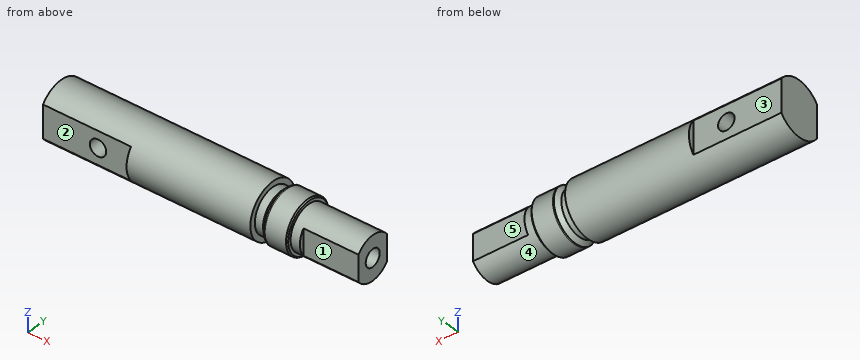
```python
from build123d import *

# Parameters (mm, degrees)
CUT_EXTRUDE1_START               = -16
CUT_EXTRUDE1_DEPTH               = 16
F_3_0MM_DOWEL_HOLE1_D            = 3
CUT_EXTRUDE3_START               = -20
SKETCH17_R                       = 5
SKETCH17_R_2                     = 4
CUT_EXTRUDE3_DEPTH               = 1.5
CHAMFER2_SIZE                    = 1
SKETCH18_R                       = 4
CUT_EXTRUDE4_DEPTH               = 3.3
TAP_DRILL_FOR_M3_HELICOIL1_D     = 3.15
TAP_DRILL_FOR_M3_HELICOIL1_DEPTH = 10
TAP_DRILL_FOR_M3_HELICOIL1_TIP   = 0.946355475
CUT_EXTRUDE5_DEPTH               = 10
SKETCH24_R                       = 5
BOSS_EXTRUDE1_DEPTH              = 3
SKETCH26_R                       = 5
SKETCH26_R_2                     = 4.7565
CUT_EXTRUDE6_DEPTH               = 0.5


# Read off the part's stored shape, not the designer's step: M10x0.75 Machine Threads Stud1
with BuildPart() as part:
    # Sketch1 → Revolve1 (revolve)
    with BuildSketch(Plane.XY, mode=Mode.PRIVATE) as revolve1_sk:
        Polygon((0, 0), (0, 5), (45, 5), (45, 4), (60, 4), (60, 0), align=None)
    revolve(revolve1_sk.sketch.rotate(Axis((0, 0, 0), (1, 0, 0)), 90), axis=Axis((0, 0, 0), (1, 0, 0)))

    # Sketch2 → Cut-Extrude1 (cut)
    with BuildSketch(Plane.ZY.offset(CUT_EXTRUDE1_START)):
        with BuildLine():
            Line((-3, 4), (3, 4))
            ThreePointArc((3, 4), (0, 5), (-3, 4))
        make_face()
        with BuildLine():
            Line((3, -4), (-3, -4))
            ThreePointArc((-3, -4), (0, -5), (3, -4))
        make_face()
    extrude(amount=CUT_EXTRUDE1_DEPTH, mode=Mode.SUBTRACT)

    # Ø3.0mm Dowel Hole1 (through all)
    with Locations(Plane(origin=(0, 4, 0), x_dir=(1, 0, 0), z_dir=(0, 1, 0))):
        with Locations((10, 0)):
            Hole(F_3_0MM_DOWEL_HOLE1_D / 2)

    # Sketch17 → Cut-Extrude3 (cut)
    with BuildSketch(Plane(origin=(60, 0, 0), x_dir=(0, 0, -1), z_dir=(1, 0, 0)).offset(CUT_EXTRUDE3_START)):
        with Locations(Location((0, 0, 0), (0, 0, 180))):
            Circle(SKETCH17_R)
        with Locations(Location((0, 0, 0), (0, 0, 180))):
            Circle(SKETCH17_R_2, mode=Mode.SUBTRACT)
    extrude(amount=-CUT_EXTRUDE3_DEPTH, mode=Mode.SUBTRACT)

    # Chamfer2
    chamfer2_edges = [part.edges().sort_by_distance(p)[0] for p in [
        (40, 0, -5),
        (45, 0, -5),
    ]]
    chamfer(chamfer2_edges, length=CHAMFER2_SIZE - 0.0001)  # a hair under: the kernel refuses the full size

    # Sketch18 → Cut-Extrude4 (cut)
    with BuildSketch(Plane(origin=(60, 0, 0), x_dir=(0, 0, -1), z_dir=(1, 0, 0))):
        with Locations(Location((0, 0, 0), (0, 0, 180))):
            Circle(SKETCH18_R)
    extrude(amount=-CUT_EXTRUDE4_DEPTH, mode=Mode.SUBTRACT)

    # Tap Drill for M3 Helicoil1
    with Locations(Plane(origin=(56.7, 0, 0), x_dir=(0, 0, -1), z_dir=(1, 0, 0))):
        with Locations((0, 0)):
            Hole(TAP_DRILL_FOR_M3_HELICOIL1_D / 2, depth=TAP_DRILL_FOR_M3_HELICOIL1_DEPTH)
            with Locations((0, 0, -(TAP_DRILL_FOR_M3_HELICOIL1_DEPTH + TAP_DRILL_FOR_M3_HELICOIL1_TIP / 2))):  # 118° drill point
                Cone(0, TAP_DRILL_FOR_M3_HELICOIL1_D / 2, TAP_DRILL_FOR_M3_HELICOIL1_TIP, mode=Mode.SUBTRACT)

    # Sketch23 → Cut-Extrude5 (cut)
    with BuildSketch(Plane(origin=(56.7, 0, 0), x_dir=(0, 0, -1), z_dir=(1, 0, 0))):
        with BuildLine():
            ThreePointArc((2.4, 3.2), (0, 4), (-2.4, 3.2))
            Line((-2.4, 3.2), (2.4, 3.2))
        make_face()
        with BuildLine():
            Line((2.4, -3.2), (-2.4, -3.2))
            ThreePointArc((-2.4, -3.2), (0, -4), (2.4, -3.2))
        make_face()
    extrude(amount=-CUT_EXTRUDE5_DEPTH, mode=Mode.SUBTRACT)

    # Sketch24 → Boss-Extrude1 (add)
    with BuildSketch(Plane(origin=(45, 0, 0), x_dir=(0, 0, -1), z_dir=(1, 0, 0))):
        Circle(SKETCH24_R)
    extrude(amount=-BOSS_EXTRUDE1_DEPTH)

    # M10x0.75 Machine Threads Stud1 outline → M10x0.75 Machine Threads Stud1 (revolve, cut)
    with BuildSketch(Plane.YX):
        Polygon((5, 45), (4.54, 45), (4.7565, 44.7835), (4.7565, 41), (5, 41), align=None)
    revolve(axis=Axis((0, 0, 0), (1, 0, 0)), mode=Mode.SUBTRACT)

    # Sketch26 → Cut-Extrude6 (cut)
    with BuildSketch(Plane(origin=(41, 0, 0), x_dir=(0, 0, -1), z_dir=(1, 0, 0))):
        with Locations(Location((0, 0, 0), (0, 0, 126.869897646))):
            Circle(SKETCH26_R)
        with Locations(Location((0, 0, 0), (0, 0, 180))):
            Circle(SKETCH26_R_2, mode=Mode.SUBTRACT)
    extrude(amount=-CUT_EXTRUDE6_DEPTH, mode=Mode.SUBTRACT)


solid = part.part
```
Here's how the part is built. I have some questions about the finished solid (model axes, mm). Face numbers are marked on the shaded views. A direction names the side the tool comes from. Give positions to 0.01 mm unless a question says otherwise; leave off trailing zeros. Loops run counter-clockwise (first coordinate to the right, second up) from the corner with the lowest first, then second, coordinate; pieces in that order, holes last. Notation, with made-up numbers: (88, 49) -> (104, 49) arc R23 cw to (104, 68) -> close; hole circle Ø7 at (79, -35.5). An arc over 180 degrees is marked (long way). Use one line per item in the form item = value. Start each with the question number.
1) Imagine slicing it at B-B (x = 48). Please give me the cut outline in (y, z) (3 decimals), then the cut area to 3 significant figures.
2) Which directions (+Z, -Z, +X, -X, +Y, -Y) give clear straight access to the entire face, cutting with the end or side of a thin tool? Please do the marked faces 1, 2, 3, 4 and 5.
3) Imagine slicing it at A-A (x = 10). Please give me the cut outline in (y, z), then the cut area to 3 significant figures.
4) Please list where these lines run through material, in increasing order: line 1 along Y through (x, z) = (54.25, 0) (3 decimals); line 2 along X through (y, z) = (-1, 0.75); line 3 along Z through (x, y) = (10, -1.5).
5) Imagine slicing it at C-C (x = 27). Please give me the cut outline in (y, z), then the cut area to 3 significant figures.
6) For P1, Ø3.5, axis at x = 10, z = 0, coming from the +Y side; P2, Ø1, axis at x = 17.5, z = -1, coming from the -Y side; P3, Ø2, axis at x = 44, z = 3, coming from the +Y side, each with a flat end and sliding along its axis, tell me the tip position at first contact or that it passes through.
Check values:
q1.outline = (-3.2, -2.4) arc R4 ccw to (3.2, -2.4) -> (3.2, 2.4) arc R4 ccw to (-3.2, 2.4) -> close; hole circle Ø3.15 at (0, 0)
q1.area = 37.2 mm^2
q2.face_1 = +Z, -Z, +X, -Y
q2.face_2 = +Z, -Z, -X, -Y
q2.face_3 = +Z, -Z, -X, +Y
q2.face_4 = +X
q2.face_5 = +Z, -Z, +X, +Y
q3.outline = (-4, -3) arc R5 ccw to (4, -3) -> (4, -1.5) -> (-4, -1.5) -> close; (-4, 1.5) -> (4, 1.5) -> (4, 3) arc R5 ccw to (-4, 3) -> close
q3.area = 46.4 mm^2
q4.line_1 = -3.2 to -1.575, 1.575 to 3.2
q4.line_2 = 0 to 8.7, 11.3 to 46.5
q4.line_3 = -4.77 to -1.5, 1.5 to 4.77
q5.outline = circle Ø10 at (0, 0)
q5.area = 78.5 mm^2
q6.P1 = 4
q6.P2 = -4.97
q6.P3 = 4.32
